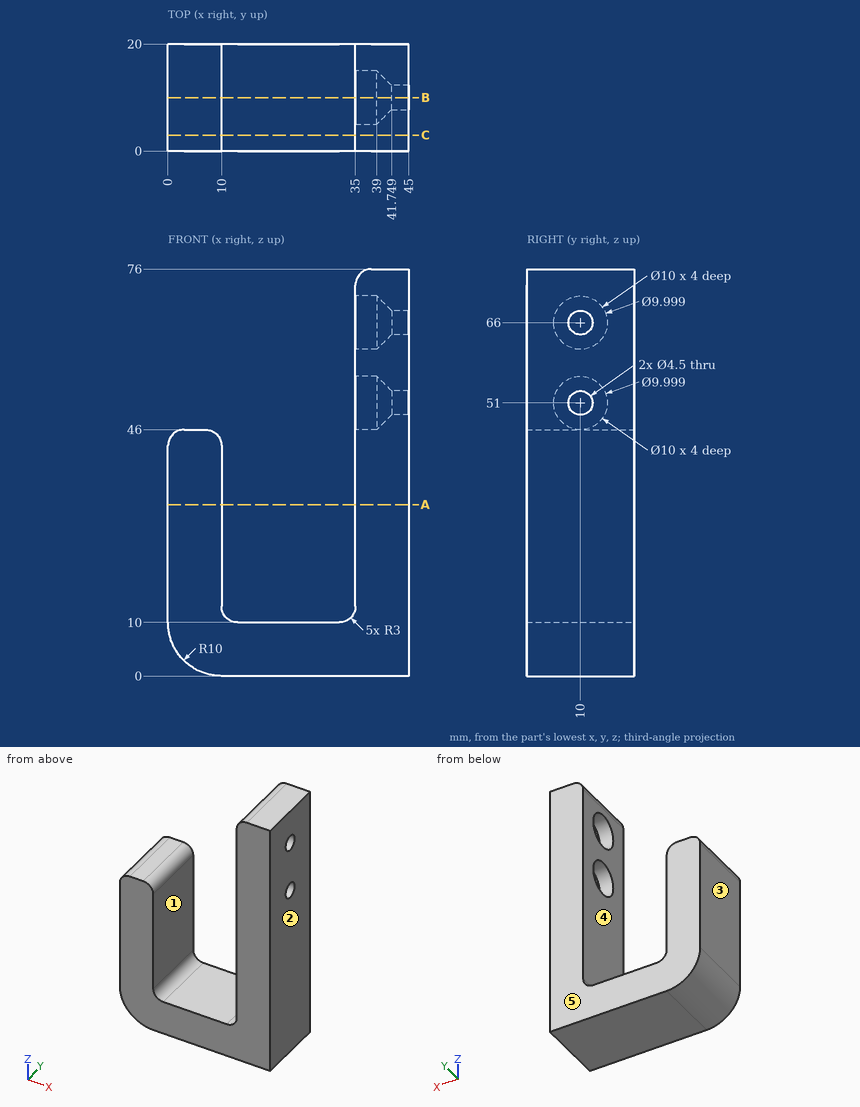
Check sheet for the drawn part. Datum: minimum x, y, z corner. Units: mm. A direction names the side the tool comes from. Round coordinates to 2 decimals unless told otherwise and drop trailing zeros. Order: outer loops, then holes, each group sorted by start corner. A loop starts at its lowest first (then second) coordinate and runs counter-clockwise, first axis right, second up. Notation, with made-up numbers: (-36, -36.75) -> (16, -36.75) arc R18 cw to (16, -21.75) -> close; hole circle Ø4 at (55.5, 17). An arc over 180 degrees is marked (long way). Return JSON: item names as keys, results as strings. Group by question number.
Q1. Release check for a two-part mould opening along X. For the marked faces 3, 4 and 5 record: released by +X, released by -X, zero draft, split by the parting line, or undercut.
Q2. Gauge pin test, flat ends, axial feed: pin 1 (8 mm diameter, centred on y = 10.5, z = 50.5, fed in from -X); pin 2 (4 mm diameter, centred on y = 10, z = 51, fed in from -X); pin 3 (7 mm diameter, centred on y = 10, z = 66, fed in from -X); pin 4 (5 mm diameter, centred on x = 18.5, y = 14, fed in from +Z). Record the tip position at first contact, or that the pin passes through.
Q3. Section check C-C, the plane y = 3. Record the boundary of the cut face in (x, z), plus the area to 3 significant figures.
Q4. Tool access check on the marked faces 1 and 2. Record the directions out of +Z, -Z, +X, -X, +Y, -Y that give a thin tool (end or side, any length) a straight path to the whole face; none if there is none.
Q5. Section check A-A, the plane z = 32. Record the boundary of the cut face in (x, y).
Q6. Section check B-B, the plane y = 10. Count the separate pieces of the cut face and the enclosed holes in it, plus the area to 3 significant figures.
Q7. Material ranges on probe 1 along Z at (x, y) = (37.05, 10) (1 decimal); probe 2 along Z at (x, y) = (35.5, 6) (1 decimal); probe 3 along X at (y, z) = (7, 27), recorded low to high. Write a range as from..to.
Numbers:
{
 "1": {"face 3": "released by -X", "face 4": "undercut", "face 5": "zero draft"},
 "2": {"pin 1": "x = 39.29", "pin 2": "through", "pin 3": "x = 40.5", "pin 4": "z = 10"},
 "3": {"outline": "(0, 10) arc R10 ccw to (10, 0) -> (45, 0) -> (45, 76) -> (38, 76) arc R3 ccw to (35, 73) -> (35, 13) arc R3 cw to (32, 10) -> (13, 10) arc R3 cw to (10, 13) -> (10, 43) arc R3 ccw to (7, 46) -> (3, 46) arc R3 ccw to (0, 43) -> close", "area": "1,450 mm^2"},
 "4": {"face 1": "+Z, +Y, -Y", "face 2": "+Z, -Z, +X, +Y, -Y"},
 "5": {"outline": "(0, 0) -> (10, 0) -> (10, 20) -> (0, 20) -> close; (35, 0) -> (45, 0) -> (45, 20) -> (35, 20) -> close"},
 "6": {"separate pieces": "3", "enclosed holes": "0", "area": "1,300 mm^2"},
 "7": {"probe 1": "0..46, 56..61, 71..75.8", "probe 2": "0..48, 54..63, 69..74.7", "probe 3": "0..10, 35..45"}
}
